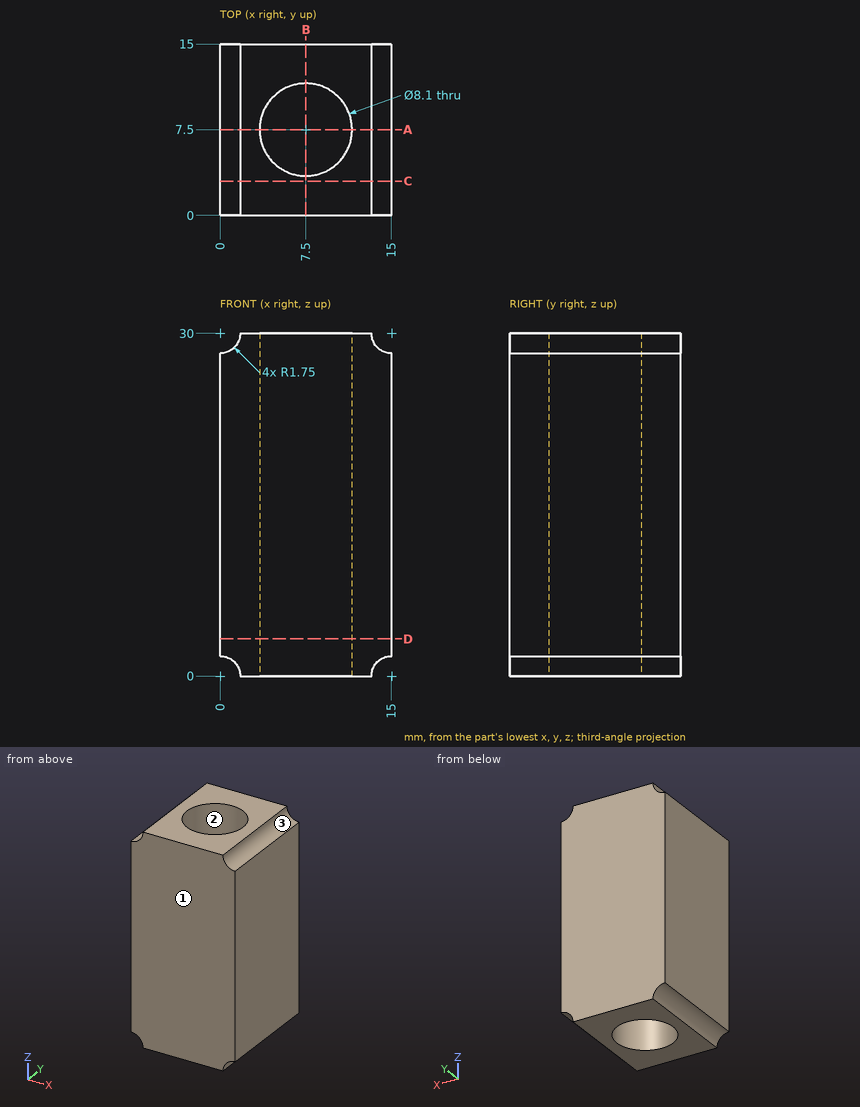
Study the drawing (mm; zero at the part's minimum x, y, z) and answer. Give positions to 0.01 mm unless a question says otherwise; leave off trailing zeros. Loops run counter-clockwise (first coordinate to the right, second up) from the corner with the lowest first, then second, coordinate; pieces in that order, holes last. Notation, with made-up numbers: (25, 60) -> (43, 60) arc R14 cw to (43, 86) -> close; hole circle Ø4 at (-36.5, -1). An arc over 180 degrees is marked (long way). Use a Markdown table: item, result. Add a question column.
1) The part is cut by section A-A, the plane y = 7.5. Determine the outline of the cut face in (x, z).
2) The part is cut by section B-B, the plane x = 7.5. Determine the outline of the cut face in (y, z), plus the area to 3 significant figures.
3) The part is cut by section C-C, the plane y = 3. Determine the outline of the cut face in (x, z).
4) Consider line 1 along Y through (x, z) = (7.5, 9.75); line 2 along Y through (x, z) = (8.5, 9.5); line 3 along X through (y, z) = (7.75, 26). Determine where each line is inside the solid, lowest interval first.
5) The part is cut by section D-D, the plane z = 3.25. Determine the outline of the cut face in (x, y), plus the area to 3 significant figures.
6) For a pull along Y with two mould halves and no side action, classify the marked faces 1, 2 and 3 as +Y half, -Y half, draft (parallel to the pull), parting line (faces both ways), or undercut.
Reported:
| question | item | result |
|---|---|---|
| 1 | outline | (0, 1.75) arc R1.75 cw to (1.75, 0) -> (3.45, 0) -> (3.45, 30) -> (1.75, 30) arc R1.75 cw to (0, 28.25) -> close; (11.55, 0) -> (13.25, 0) arc R1.75 cw to (15, 1.75) -> (15, 28.25) arc R1.75 cw to (13.25, 30) -> (11.55, 30) -> close |
| 2 | outline | (0, 0) -> (3.45, 0) -> (3.45, 30) -> (0, 30) -> close; (11.55, 0) -> (15, 0) -> (15, 30) -> (11.55, 30) -> close |
| 2 | area | 207 mm^2 |
| 3 | outline | (0, 1.75) arc R1.75 cw to (1.75, 0) -> (13.25, 0) arc R1.75 cw to (15, 1.75) -> (15, 28.25) arc R1.75 cw to (13.25, 30) -> (1.75, 30) arc R1.75 cw to (0, 28.25) -> close |
| 4 | line 1 | y = 0 to 3.45, 11.55 to 15 |
| 4 | line 2 | y = 0 to 3.58, 11.42 to 15 |
| 4 | line 3 | x = 0 to 3.46, 11.54 to 15 |
| 5 | outline | (0, 0) -> (15, 0) -> (15, 15) -> (0, 15) -> close; hole circle Ø8.1 at (7.5, 7.5) |
| 5 | area | 173 mm^2 |
| 6 | face 1 | -Y half |
| 6 | face 2 | undercut |
| 6 | face 3 | draft |
